Can you work these out from the model? Positions are in its coordinate system, mm. A direction names the side the tool comes from. Give positions to 0.01 mm unless a question says otherwise; leave off trailing zeros. Write each loop counter-clockwise with the first axis right and the second up, starting at its lowest first coordinate (ties: lowest second). Pieces come first, ordered by that corner, then holes. Notation, with made-up numbers: M 35,-4 L 60,-4 A19 ccw 60,13 Z; hole C -28.75,82 d10. An arc over 180 degrees is marked long. Write each question's results on one line, items separated by ' | '.
from build123d import *

# Parameters (mm, degrees)
SKETCH2_W          = 5
SKETCH2_H          = 4.464495409
CUT_EXTRUDE1_DEPTH = 82.228385508
FILLET1_R          = 2
FILLET2_R          = 2


with BuildPart() as part:
    # Sketch1 → Revolve1 (revolve)
    with BuildSketch(Plane.XY, mode=Mode.PRIVATE) as revolve1_sk:
        Polygon((-12.114285714, 13.542857143), (11.885714286, 13.542857143), (11.885714286, 9.542857143), (4, 9.542857143), (4, -14.457142857), (11.885714286, -14.457142857), (11.885714286, -18.457142857), (-12.114285714, -18.457142857), (-12.114285714, -14.457142857), (-4, -14.457142857), (-4, 9.542857143), (-12.114285714, 9.542857143), (-12.114285714, 12.742857143), align=None)
    revolve(revolve1_sk.sketch.rotate(Axis((-20.457142857, -26.457142857, 0), (1, 0, 0)), 90), axis=Axis((-20.457142857, -26.457142857, 0), (1, 0, 0)))

    # Sketch2 → Cut-Extrude1 (cut, through all)
    with BuildSketch(Plane(origin=(12, 0, 0), x_dir=(0, 0, -1), z_dir=(1, 0, 0))):
        with Locations((0, -18.189390562)):
            Rectangle(SKETCH2_W, SKETCH2_H)
    extrude(amount=-CUT_EXTRUDE1_DEPTH, mode=Mode.SUBTRACT)

    # Fillet1
    fillet1_edges = [part.edges().sort_by_distance(p)[0] for p in [
        (4, -26.457142857, -12),
    ]]
    fillet(fillet1_edges, radius=FILLET1_R)

    # Fillet2
    fillet2_edges = [part.edges().sort_by_distance(p)[0] for p in [
        (-4, -26.457142857, -12),
    ]]
    fillet(fillet2_edges, radius=FILLET2_R)


solid = part.part
Item 1: I'm going to push flat-ended pins straight in: pin 1 (1.5 mm diameter, centred on x = -2.5, y = -17.5, fed in from +Z); pin 2 (1 mm diameter, centred on y = -47.5, z = -13, fed in from +X); pin 3 (12 mm diameter, centred on y = -49.5, z = -6.5, fed in from -X); pin 4 (8 mm diameter, centred on y = -54.5, z = 31, fed in from +X). Where does each tip first touch, or does it pass through?
Geometry says:
pin 1: stops at z = 39.15 | pin 2: stops at x = 4 | pin 3: stops at x = -4 | pin 4: stops at x = 11.89
Item 2: I want a section at B-B, the plane x = -9.5. Please give me the cut outline in (y, z), and give its area (3 significant figures).
Geometry says:
outline: C -26.46,0 d80; C -26.46,0 d24; hole C -26.46,0 d72; hole M -18.86,-2.5 L -15.96,-2.5 L -15.96,2.5 L -18.86,2.5 A8 ccw long Z | area: 1,190 mm2
Item 3: I want a section at C-C, the plane z = 26.5. Please give me the cut outline in (x, y), and give its area (3 significant figures).
Geometry says:
outline: M -12.11,-56.42 L 11.89,-56.42 L 11.89,-50.82 L 4,-50.82 L 4,-2.09 L 11.89,-2.09 L 11.89,3.51 L -12.11,3.51 L -12.11,-2.09 L -4,-2.09 L -4,-50.82 L -12.11,-50.82 Z | area: 658 mm2
Item 4: For faces 4 (the face through (4, -11, -1)), 5 (the face through (0, -17, -2.5)), 6 (the face through (-9.014, -14.742, -2.601)), which set-ups out of +Z, -Z, +X, -X, +Y, -Y let a thin tool reach every point of the face, with its end or its side?
Geometry says:
face 4: +X | face 5: +X, -X | face 6: -X
Item 5: I want a section at D-D, the plane y = -5.5. Please give me the cut outline in (x, z).
Geometry says:
outline: M -12.11,-34.07 L 11.89,-34.07 L 11.89,-29.27 L 4,-29.27 L 4,29.27 L 11.89,29.27 L 11.89,34.07 L -12.11,34.07 L -12.11,29.27 L -4,29.27 L -4,-29.27 L -12.11,-29.27 Z
Item 6: I want a section at A-A, the plane z = 0. Please give me the cut outline in (x, y), and give its area (3 significant figures).
Geometry says:
outline: M -12.11,-66.46 L 11.89,-66.46 L 11.89,-62.46 L 4,-62.46 L 4,-40.46 A2 cw 6,-38.46 L 11.89,-38.46 L 11.89,-34.46 L -12.11,-34.46 L -12.11,-38.46 L -6,-38.46 A2 cw -4,-40.46 L -4,-62.46 L -12.11,-62.46 Z; M -12.11,-15.96 L 11.89,-15.96 L 11.89,-14.46 L 6,-14.46 A2 cw 4,-12.46 L 4,9.54 L 11.89,9.54 L 11.89,13.54 L -12.11,13.54 L -12.11,9.54 L -4,9.54 L -4,-12.46 A2 cw -6,-14.46 L -12.11,-14.46 Z | area: 711 mm2
Item 7: Thinking about a two-plate mould opening in Y: for faces 1 (the face through (0.05, -53.49, -29.48)), 2 (the face through (8.984, -14.742, -2.601)), 3 (the face through (-12.114, -35, 0)), which applies, +Y half, -Y half, draft (parallel to the pull), parting line (faces both ways), or undercut?
Geometry says:
face 1: parting line | face 2: undercut | face 3: draft
Item 8: If I drill on line 1 (Y direction, x = -6.75, z = 0); line 2 (Z direction, x = 6.75, y = -23); line 3 (Y direction, x = -5, z = 0), over which ranges is the centre line in solid material (lowest first)? Write a range as from..to.
Geometry says:
line 1: y = -66.46..-62.46, -38.46..-34.46, -15.96..-14.46, 9.54..13.54 | line 2: z = -39.85..-35.83, -11.49..-7.21, 7.21..11.49, 35.83..39.85 | line 3: y = -66.46..-62.46, -38.73..-34.46, -15.96..-14.19, 9.54..13.54
